Drawing for the job (mm, zero at the part's lowest x, y, z). A direction names the side the tool comes from. Give positions to 0.01 mm unless a question says otherwise; leave off trailing zeros. Write each loop counter-clockwise with the first axis right and the second up, starting at its lowest first coordinate (ties: lowest second). Pieces come first, ordered by that corner, then holes. Notation, with made-up numbers: M 80,-32.75 L 91,-32.75 A14 ccw 91,-13.75 Z; hole C -6,79 d11. An arc over 180 degrees is marked long. Answer as a JSON object with one key per item and string values. Group by question number.
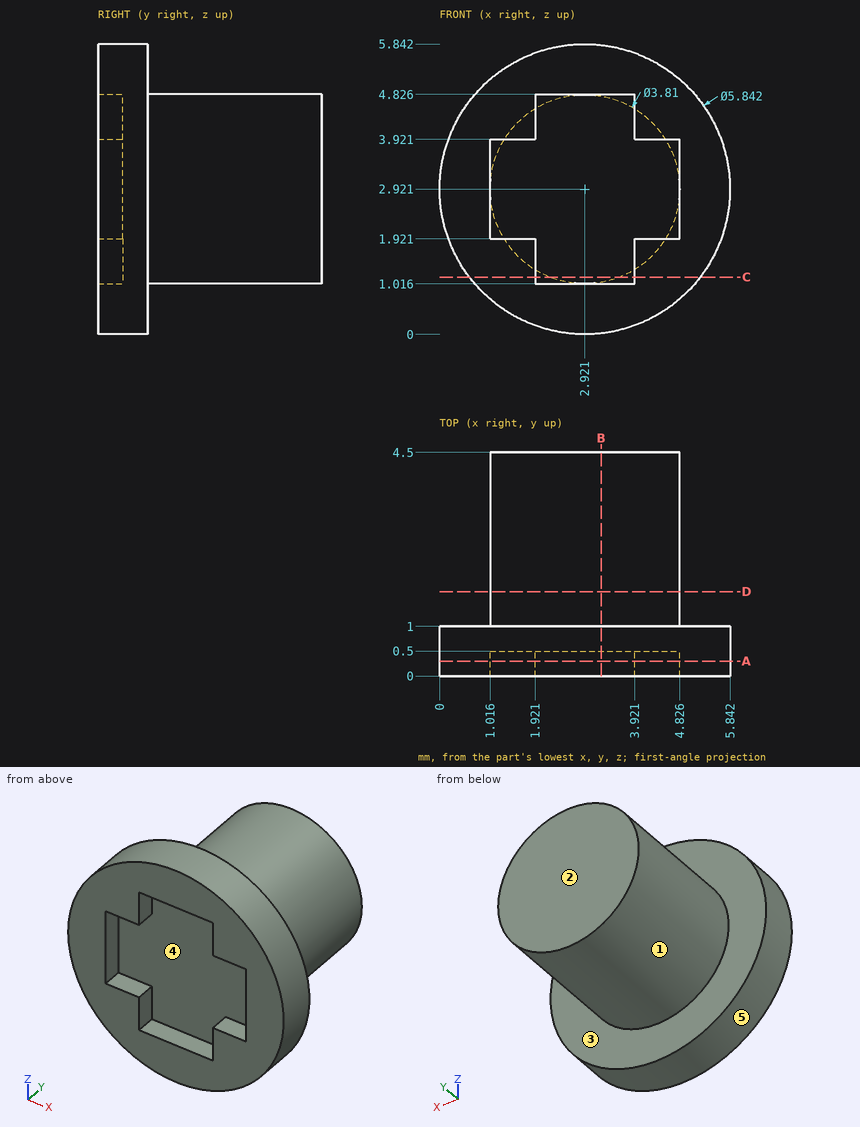
Q1. Slice it at A-A, the plane y = 0.3. Write the cut outline in (x, z), then the cut area to 3 significant figures.
Q2. 3-axis set-ups, long thin cutter, end or side, ignore diameter. For the marked faces 1 and 2: which of +Z, -Z, +X, -X, +Y, -Y reach the whole face in a straight line?
Q3. Drop flat-ended pins along their axis: P1, Ø1, axis at x = 2.5, y = 2.5, coming from the -Z side; P2, Ø1.1, axis at x = 2.5, z = 3, coming from the -Y side; P3, Ø1.5, axis at x = 4.5, y = 0.5, coming from the +Z side. Give the stop position or say it passes through.
Q4. Wall check: L1, parallel to Z at x = 2.9, y = 1.3; L2, parallel to Y at x = 4.6, z = 0.65; L3, parallel to Z at x = 1.3, y = 0.3. Give the ranges that are in metal, low to high.
Q5. Two-plate mould, pull along Z, no slides. Class the marked faces 3, 4 and 5: +Z half, -Z half, draft (parallel to the pull), parting line (faces both ways), or undercut.
Q6. Slice it at B-B, the plane x = 3.25. Write the cut outline in (y, z).
Q7. Slice it at C-C, the plane z = 1.15. Write the cut outline in (x, y).
Q8. Slice it at D-D, the plane y = 1.7. Write the cut outline in (x, z) (3 decimals), then the cut area to 3 significant figures.
Solved:
{
 "1": {"outline": "C 2.92,2.92 d5.84; hole M 1.02,1.92 L 1.92,1.92 L 1.92,1.02 L 3.92,1.02 L 3.92,1.92 L 4.83,1.92 L 4.83,3.92 L 3.92,3.92 L 3.92,4.83 L 1.92,4.83 L 1.92,3.92 L 1.02,3.92 Z", "area": "15.6 mm²"},
 "2": {"face 1": "+Y", "face 2": "+Z, -Z, +X, -X, +Y"},
 "3": {"P1": "stops at z = 1.02", "P2": "stops at y = 0.5", "P3": "stops at z = 5.72"},
 "4": {"L1": "z = 1.02 to 4.83", "L2": "y = 0 to 1", "L3": "z = 0.49 to 1.92, 3.92 to 5.35"},
 "5": {"face 3": "draft", "face 4": "undercut", "face 5": "parting line"},
 "6": {"outline": "M 0,0.02 L 1,0.02 L 1,1.04 L 4.5,1.04 L 4.5,4.8 L 1,4.8 L 1,5.82 L 0,5.82 L 0,4.83 L 0.5,4.83 L 0.5,1.02 L 0,1.02 Z"},
 "7": {"outline": "M 0.6,0 L 1.92,0 L 1.92,0.5 L 3.92,0.5 L 3.92,0 L 5.24,0 L 5.24,1 L 3.62,1 L 3.62,4.5 L 2.22,4.5 L 2.22,1 L 0.6,1 Z"},
 "8": {"outline": "C 2.921,2.921 d3.81", "area": "11.4 mm²"}
}
